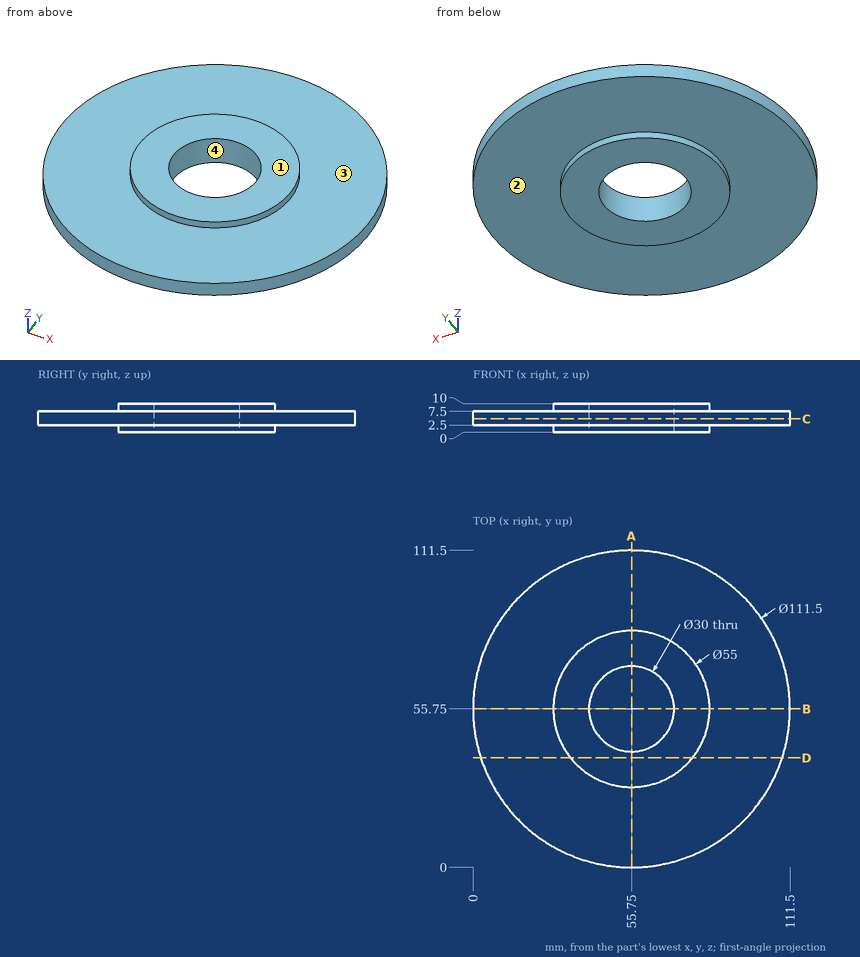
Drawing for the job (mm, zero at the part's lowest x, y, z). A direction names the side the tool comes from. Coordinates: 2 decimals unless noted, no trailing zeros. Order: outer loops, then holes, each group sorted by start corner. A loop starts at its lowest first (then second) coordinate and runs counter-clockwise, first axis right, second up. Notation, with made-up numbers: (34.25, 27) -> (84.25, 27) arc R25 cw to (84.25, 59) -> close; hole circle Ø2 at (-11.5, 45). An arc over 180 degrees is marked (long way). Answer in a Markdown table with one row per item.
1) Band-saw the part on C-C (z = 4.75). List the corners of the cut face in (x, y).
Check values:
| item | result |
|---|---|
| outline | circle Ø111.5 at (55.75, 55.75); hole circle Ø30 at (55.75, 55.75) |
2) Which spindle directions (+Z, -Z, +X, -X, +Y, -Y) get a long thin tool onto all of the face, cutting with end or side? Do the marked faces 1 and 2. Say none if no direction does.
Check values:
| item | result |
|---|---|
| face 1 | +Z, +X, -X, +Y, -Y |
| face 2 | -Z |
3) Drill centre lines: line 1 (Y direction, x = 55.75, z = 3.75); line 2 (Z direction, x = 88, y = 68); line 3 (Y direction, x = 69, z = 1.25). Where is each one in solid material? Low to high.
Check values:
| item | result |
|---|---|
| line 1 | 0 to 40.75, 70.75 to 111.5 |
| line 2 | 2.5 to 7.5 |
| line 3 | 31.65 to 48.72, 62.78 to 79.85 |
4) Band-saw the part on D-D (y = 38.5). List the corners of the cut face in (x, z).
Check values:
| item | result |
|---|---|
| outline | (2.74, 2.5) -> (34.33, 2.5) -> (34.33, 0) -> (77.17, 0) -> (77.17, 2.5) -> (108.76, 2.5) -> (108.76, 7.5) -> (77.17, 7.5) -> (77.17, 10) -> (34.33, 10) -> (34.33, 7.5) -> (2.74, 7.5) -> close |
5) Mould opens along Y. For the marked faces 3 and 4 say: pulls with the +Y half, pulls with the -Y half, needs draft (parallel to the pull), parting line crosses it, or undercut.
Check values:
| item | result |
|---|---|
| face 3 | needs draft |
| face 4 | undercut |
6) Band-saw the part on A-A (x = 55.75). List the corners of the cut face in (y, z), and give its area (4 significant figures).
Check values:
| item | result |
|---|---|
| outline | (0, 2.5) -> (28.25, 2.5) -> (28.25, 0) -> (40.75, 0) -> (40.75, 10) -> (28.25, 10) -> (28.25, 7.5) -> (0, 7.5) -> close; (70.75, 0) -> (83.25, 0) -> (83.25, 2.5) -> (111.5, 2.5) -> (111.5, 7.5) -> (83.25, 7.5) -> (83.25, 10) -> (70.75, 10) -> close |
| area | 532.5 mm2 |
7) Flat gauge pins, fed straight in: P1, Ø5, axis at y = 67, z = 6, coming from the +X side; P2, Ø4, axis at y = 40, z = 7, coming from the -X side; P3, Ø4, axis at y = 92.5, z = 2, coming from the +X side; P4, Ø12, axis at x = 63, y = 27, coming from the -Z side. Where does each tip first touch, or does it go through?
Check values:
| item | result |
|---|---|
| P1 | x = 110.81 |
| P2 | x = 1.72 |
| P3 | x = 99.29 |
| P4 | z = 0 |
